Verification items for the finished model (mm, model axes). Face numbers are marked on the shaded views. A direction names the side the tool comes from. Give positions to 0.01 mm unless a question says otherwise; leave off trailing zeros. Write each loop counter-clockwise with the first axis right and the second up, starting at its lowest first coordinate (ties: lowest second). Pieces come first, ordered by that corner, then holes.
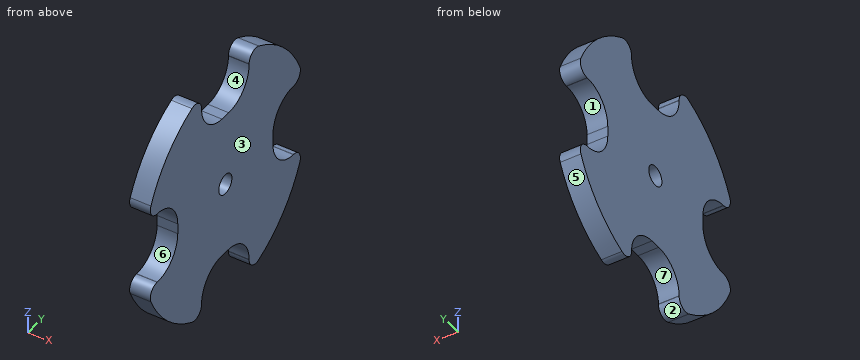
from build123d import *

# Parameters (mm, degrees)
SKETCH1_R           = 0.965
BOSS_EXTRUDE1_DEPTH = 2
CUT_EXTRUDE1_DEPTH  = 18.088007491
CIRPATTERN3_COUNT   = 4
FILLET5_R           = 1


with BuildPart() as part:
    # Sketch1 → Boss-Extrude1 (new body)
    # profile 1 of 2: a face of its own
    with BuildSketch(Plane(origin=(0, 0, 0), x_dir=(0, 0, -1), z_dir=(1, 0, 0))):
        with BuildLine():
            ThreePointArc((-0.5, 7), (-2.621320344, 7.878679656), (-3.5, 10))
            Line((-3.5, 10), (-3.5, 11.478240283))
            ThreePointArc((-3.5, 11.478240283), (-7.141428429, -9.643650761), (12, 0))
            ThreePointArc((12, 0), (9.643650761, 7.141428429), (3.5, 11.478240283))
            Line((3.5, 11.478240283), (3.5, 10))
            ThreePointArc((3.5, 10), (2.621320344, 7.878679656), (0.5, 7))
            Line((0.5, 7), (-0.5, 7))
        make_face()
        Circle(SKETCH1_R, mode=Mode.SUBTRACT)
    # profile 2 of 2: a face of its own
    with BuildSketch(Plane(origin=(0, 0, 0), x_dir=(0, 0, -1), z_dir=(1, 0, 0))):
        with BuildLine():
            Line((-3.5, 11.478240283), (-3.5, 10))
            ThreePointArc((-3.5, 10), (-2.621320344, 7.878679656), (-0.5, 7))
            Line((-0.5, 7), (0.5, 7))
            ThreePointArc((0.5, 7), (2.621320344, 7.878679656), (3.5, 10))
            Line((3.5, 10), (3.5, 11.478240283))
            ThreePointArc((3.5, 11.478240283), (0, 12), (-3.5, 11.478240283))
        make_face()
    extrude(amount=BOSS_EXTRUDE1_DEPTH)

    # Sketch1_3 → Cut-Extrude1 (cut, through all)
    with BuildSketch(Plane(origin=(0, 0, 0), x_dir=(0, 0, -1), z_dir=(1, 0, 0))):
        with BuildLine():
            Line((-3.5, 11.478240283), (-3.5, 10))
            ThreePointArc((-3.5, 10), (-2.621320344, 7.878679656), (-0.5, 7))
            Line((-0.5, 7), (0.5, 7))
            ThreePointArc((0.5, 7), (2.621320344, 7.878679656), (3.5, 10))
            Line((3.5, 10), (3.5, 11.478240283))
            ThreePointArc((3.5, 11.478240283), (0, 12), (-3.5, 11.478240283))
        make_face()
    cut_extrude1 = extrude(amount=CUT_EXTRUDE1_DEPTH, mode=Mode.SUBTRACT)

    # CirPattern3: Cut-Extrude1 ×4 about axis
    cirpattern3_axis = Axis((0, 0, 0), (1, 0, 0))
    for i in range(1, CIRPATTERN3_COUNT):
        add(cut_extrude1.rotate(cirpattern3_axis, i * 360 / CIRPATTERN3_COUNT), mode=Mode.SUBTRACT)

    # Fillet5
    fillet5_edges = [part.edges().sort_by_distance(p)[0] for p in [
        (1, 11.478240283, -3.5),
        (1, 11.478240283, 3.5),
        (1, -3.5, -11.478240283),
        (1, 3.5, -11.478240283),
        (1, -11.478240283, 3.5),
        (1, -11.478240283, -3.5),
        (1, 3.5, 11.478240283),
        (1, -3.5, 11.478240283),
    ]]
    fillet(fillet5_edges, radius=FILLET5_R)


solid = part.part
Item 1: Depth check by flat-ended pin: pin 1 (0.5 mm diameter, centred on x = 1, y = 0, fed in from +Z); pin 2 (1.7 mm diameter, centred on y = 0, z = 0, fed in from -X); pin 3 (1.1 mm diameter, centred on x = 1, z = 0, fed in from -Y); pin 4 (1.1 mm diameter, centred on x = 1, y = 0, fed in from -Z). Enter the tip coordinate at first touch or a pass-through.
Answer key:
pin 1: stops at z = 7
pin 2: passes through
pin 3: stops at y = -7
pin 4: stops at z = -7
Item 2: Set-up check for the marked faces 5, 6 and 7: record each of +Z, -Z, +X, -X, +Y, -Y from which the full face is reachable in a straight line by a thin tool's end or side.
Answer key:
face 5: -Z, +X, -X, +Y
face 6: +X, -X, -Y
face 7: -Z, +X, -X
Item 3: Scan lines: line 1 along Y through (x, z) = (1.15, 0) (3 decimals); line 2 along Y through (x, z) = (0.65, -9.25); line 3 along Z through (x, y) = (1.45, 10.25). Record each from-to range of solid material in increasing order.
Answer key:
line 1: y = -7 to -0.965, 0.965 to 7
line 2: y = -7.64 to -3.4, 3.4 to 7.64
line 3: z = -6.24 to -3.52, 3.52 to 6.24
Item 4: Release check for a two-part mould opening along Z. For the marked faces 1, 2, 3 and 4 record: released by +Z, released by -Z, zero draft, split by the parting line, or undercut.
Answer key:
face 1: undercut
face 2: released by -Z
face 3: zero draft
face 4: released by +Z
Item 5: Sectioned sample at D-D on z = -5.25. Record the cut outline in (x, y), then the cut area to 3 significant figures.
Answer key:
outline: (0, -10.79) - (2, -10.79) - (2, 10.79) - (0, 10.79) - close
area: 43.2 mm2
Item 6: Sectioned sample at A-A on z = 0. Record the cut outline in (x, y) (3 decimals), then the cut area to 3 significant figures.
Answer key:
outline: (0, -7) - (2, -7) - (2, -0.965) - (0, -0.965) - close; (0, 0.965) - (2, 0.965) - (2, 7) - (0, 7) - close
area: 24.1 mm2
